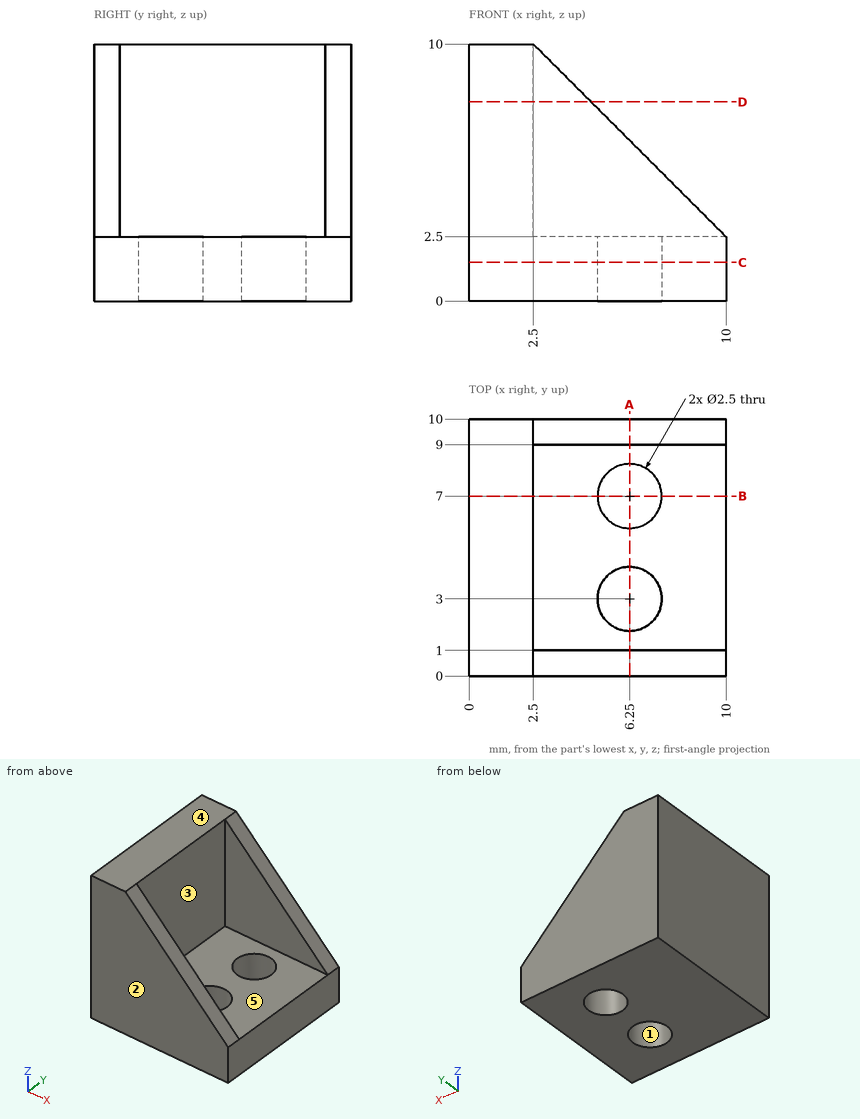
Geometry check sheet. Reference: drawing and pictorial views, mm from the part's lowest x, y, z. A direction names the side the tool comes from. Coordinates: 2 decimals unless noted, no trailing zeros. Order: outer loops, then holes, each group sorted by start corner. A loop starts at its lowest first (then second) coordinate and runs counter-clockwise, first axis right, second up. Notation, with made-up numbers: (13.5, 83) -> (70.5, 83) arc R15 cw to (70.5, 90) -> close; hole circle Ø1 at (18.5, 72). An arc over 180 degrees is marked (long way). Put each result on its own line as item: value. Start each with the question number.
1) Cross-section at C-C (z = 1.5). Enter the section's corners in (x, y), plus the area to 3 significant figures.
2) Cross-section at D-D (z = 7.75). Enter the section's corners in (x, y).
3) Material ranges on L1, parallel to Y at x = 6.25, z = 1.45; L2, parallel to X at y = 3, z = 1.05; L3, parallel to Y at x = 5.25, z = 2, recorded low to high.
4) Tool access check on the marked faces 4 and 5. Record the directions out of +Z, -Z, +X, -X, +Y, -Y that give a thin tool (end or side, any length) a straight path to the whole face; none if there is none.
5) Go/stop test with flat-tipped pins: pin 1 (2 mm diameter, centred on x = 4.5, y = 6, fed in from +Z); pin 2 (4 mm diameter, centred on x = 1, y = 7, fed in from -Z); pin 3 (2 mm diameter, centred on y = 5.5, z = 5, fed in from +X); pin 4 (1.5 mm diameter, centred on x = 6.25, y = 3, fed in from -Z). Record where each tip stops, or that it passes through.
6) Release check for a two-part mould opening along X. For the marked faces 1, 2 and 3 record: pulls with the +X half, pulls with the -X half, needs draft (parallel to the pull), parting line crosses it, or undercut.
7) Cross-section at B-B (y = 7). Enter the section's corners in (x, z).
8) Cross-section at A-A (x = 6.25). Enter the section's corners in (y, z).
Geometry check:
1. outline: (0, 0) -> (10, 0) -> (10, 10) -> (0, 10) -> close; hole circle Ø2.5 at (6.25, 3); hole circle Ø2.5 at (6.25, 7)
1. area: 90.2 mm^2
2. outline: (0, 0) -> (4.75, 0) -> (4.75, 1) -> (2.5, 1) -> (2.5, 9) -> (4.75, 9) -> (4.75, 10) -> (0, 10) -> close
3. L1: y = 0 to 1.75, 4.25 to 5.75, 8.25 to 10
3. L2: x = 0 to 5, 7.5 to 10
3. L3: y = 0 to 2.25, 3.75 to 6.25, 7.75 to 10
4. face 4: +Z, +X, -X, +Y, -Y
4. face 5: +Z, +X
5. pin 1: stops at z = 2.5
5. pin 2: stops at z = 0
5. pin 3: stops at x = 2.5
5. pin 4: passes through
6. face 1: undercut
6. face 2: needs draft
6. face 3: pulls with the +X half
7. outline: (0, 0) -> (5, 0) -> (5, 2.5) -> (2.5, 2.5) -> (2.5, 10) -> (0, 10) -> close; (7.5, 0) -> (10, 0) -> (10, 2.5) -> (7.5, 2.5) -> close
8. outline: (0, 0) -> (1.75, 0) -> (1.75, 2.5) -> (1, 2.5) -> (1, 6.25) -> (0, 6.25) -> close; (4.25, 0) -> (5.75, 0) -> (5.75, 2.5) -> (4.25, 2.5) -> close; (8.25, 0) -> (10, 0) -> (10, 6.25) -> (9, 6.25) -> (9, 2.5) -> (8.25, 2.5) -> close
